CAD build for the part. Positions are in the model's coordinates, mm. A direction names the side the tool comes from. Round coordinates to 2 decimals unless told otherwise and drop trailing zeros. Loops run counter-clockwise (first coordinate to the right, second up) from the corner with the lowest first, then second, coordinate; pieces in that order, holes last. Notation, with made-up numbers: (37, 72.25) - (64, 72.25) arc R10 ccw to (64, 83.25) - close; hole circle Ø4 at (10, 59). An arc over 180 degrees is marked (long way). One line per question, with ' | ' between items.
```python
from build123d import *

# Parameters (mm, degrees)
F0_R     = 11.6205
F1_DEPTH = 18.7452
F2_R     = 2.54
F3_DEPTH = 10.922
F4_SIZE  = 3.81
F5_SIZE  = 1.27
F6_W     = 5.842
F6_H     = 20.32
F7_DEPTH = 2.794


with BuildPart() as f1:
    # F0 (on Top) → F1 (new body)
    with BuildSketch(Plane.XY):
        Circle(F0_R)
    extrude(amount=F1_DEPTH)

    # F2 (on face) → F3 (join)
    with BuildSketch(Plane.XY.offset(18.7452)):
        Circle(F2_R)
    extrude(amount=F3_DEPTH)

    # F4
    f4_edges = [f1.edges().sort_by_distance(p)[0] for p in [
        (-11.6205, 0, 18.7452),
    ]]
    chamfer(f4_edges, length=F4_SIZE)

    # F5
    f5_edges = [f1.edges().sort_by_distance(p)[0] for p in [
        (-11.6205, 0, 0),
    ]]
    chamfer(f5_edges, length=F5_SIZE)

    # F6 (on face) → F7 (join)
    with BuildSketch(Plane(origin=(0, 0, 0), x_dir=(1, 0, 0), z_dir=(0, 0, -1))):
        with Locations((0, 10.16)):
            Rectangle(F6_W, F6_H)
    extrude(amount=-F7_DEPTH)


solid = f1.part
```
(1) Cut at B-B, the plane x = 0. Write the cut outline in (y, z).
Results found:
outline: (-20.32, 0) - (10.35, 0) - (11.62, 1.27) - (11.62, 14.94) - (7.81, 18.75) - (2.54, 18.75) - (2.54, 29.67) - (-2.54, 29.67) - (-2.54, 18.75) - (-7.81, 18.75) - (-11.62, 14.94) - (-11.62, 2.79) - (-20.32, 2.79) - close
(2) Drop flat-ended pins along their axis: P1, Ø2, axis at x = 7, z = 10.5, coming from the +Y side; P2, Ø4, axis at x = -6, z = 13.5, coming from the +Y side; P3, Ø4, axis at y = -5, z = 18.5, coming from the -X side. Give the stop position or say it passes through.
Results found:
P1: stops at y = 9.95 | P2: stops at y = 10.91 | P3: stops at x = -8.95
(3) Tool access for faces 1 (the face through (0, -20.32, 1)), 2 (the face through (-0.33, 2.52, 24.13)): list every direction of +Z, -Z, +X, -X, +Y, -Y with a clear straight run to the whole face (end or side of a thin tool).
Results found:
face 1: +Z, -Z, +X, -X, -Y | face 2: +Z
(4) Cut at C-C, the plane z = 7. Write the cut outline in (x, y), then the cut area to 3 significant figures.
Results found:
outline: circle Ø23.24 at (0, 0) | area: 424 mm²
(5) Cut at D-D, the plane y = -14. Write the cut outline in (x, z).
Results found:
outline: (-2.92, 0) - (2.92, 0) - (2.92, 2.79) - (-2.92, 2.79) - close
(6) Probe L1, parallel to Z at x = 2.75, y = -18.5; L2, parallel to Z at x = 3, y = -0.5; L3, parallel to Y at x = -0.25, z = 1.5. List the from-to ranges inside material, lowest first.
Results found:
L1: z = 0 to 2.79 | L2: z = 0 to 18.75 | L3: y = -20.32 to 11.62
(7) Cut at A-A, the plane y = 0. Write the cut outline in (x, z), then the cut area to 3 significant figures.
Results found:
outline: (-11.62, 1.27) - (-10.35, 0) - (10.35, 0) - (11.62, 1.27) - (11.62, 14.94) - (7.81, 18.75) - (2.54, 18.75) - (2.54, 29.67) - (-2.54, 29.67) - (-2.54, 18.75) - (-7.81, 18.75) - (-11.62, 14.94) - close | area: 475 mm²
